Verification items for this drawing (mm, ordinates from the low corner). A direction names the side the tool comes from. Give positions to 0.01 mm unless a question says otherwise; leave off trailing zeros. Loops run counter-clockwise (first coordinate to the right, second up) from the corner with the lowest first, then second, coordinate; pieces in that order, holes last. Notation, with made-up numbers: (40.25, 65.5) -> (72.25, 65.5) arc R6 cw to (72.25, 73.5) -> close; hole circle Ø2 at (20.25, 49). An arc over 180 degrees is marked (long way). Answer as a JSON object with one key per item and string values.
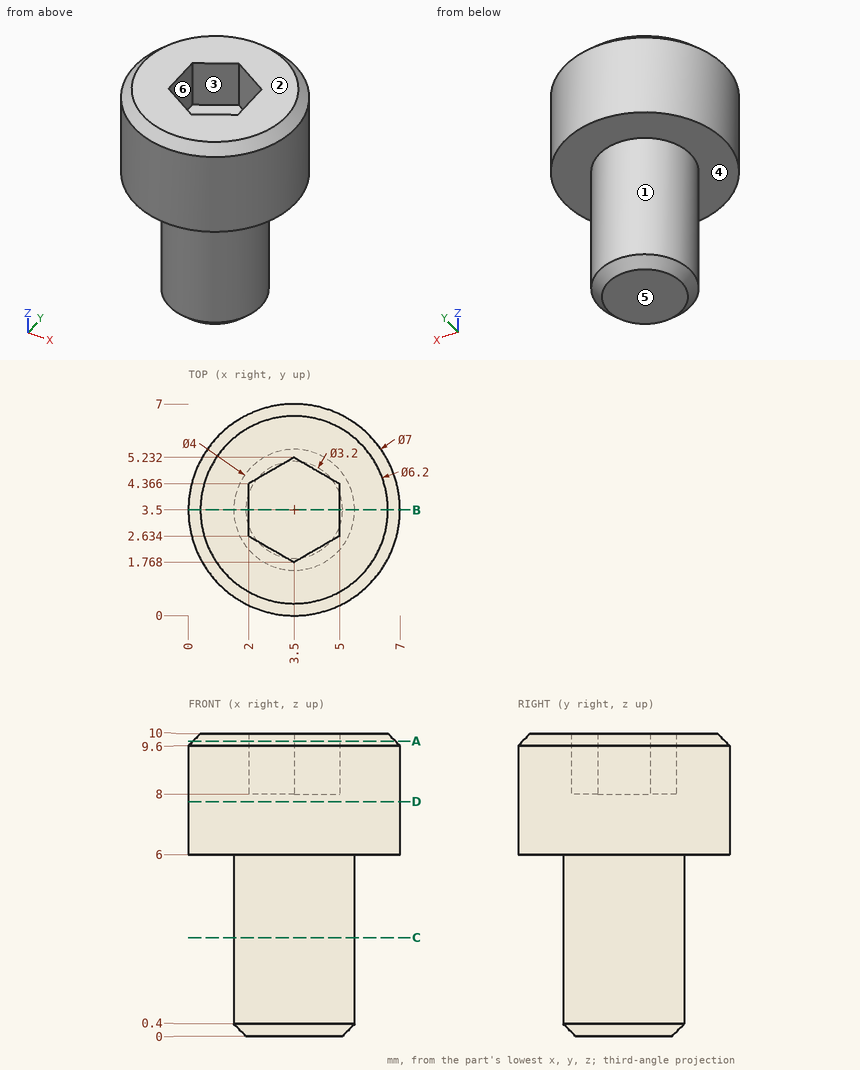
1) Draft check along X on the marked faces 1, 2 and 3. Enter one of: pulls with the +X half, pulls with the -X half, needs draft (parallel to the pull), parting line crosses it, or undercut.
Geometry check:
{"face 1": "parting line crosses it", "face 2": "needs draft", "face 3": "undercut"}
2) Section check C-C on z = 3.25. Record the cut outline in (x, y).
Geometry check:
{"outline": "circle Ø4 at (3.5, 3.5)"}
3) Depth check by flat-ended pin: P1, Ø0.5, axis at y = 4, z = 9, coming from the -X side; P2, Ø3, axis at x = 3, y = 5, coming from the -Z side; P3, Ø2, axis at x = 5.5, z = 9, coming from the -Y side. Enter the tip coordinate at first touch or a pass-through.
Geometry check:
{"P1": "stops at x = 0.01", "P2": "stops at z = 0", "P3": "stops at y = 0.15"}
4) Section check A-A on z = 9.75. Record the cut outline in (x, y).
Geometry check:
{"outline": "circle Ø6.7 at (3.5, 3.5); hole (2, 2.63) -> (3.5, 1.77) -> (5, 2.63) -> (5, 4.37) -> (3.5, 5.23) -> (2, 4.37) -> close"}
5) Tool access check on the marked faces 4, 5 and 6. Record the directions out of +Z, -Z, +X, -X, +Y, -Y that give a thin tool (end or side, any length) a straight path to the whole face; none if there is none.
Geometry check:
{"face 4": "-Z", "face 5": "-Z, +X, -X, +Y, -Y", "face 6": "+Z"}
6) Material ranges on line 1 along Z through (x, y) = (4, 6.25); line 2 along Y through (x, z) = (3.5, 3.25); line 3 along Z through (x, y) = (4.5, 4.5), recorded low to high. Write a range as from..to.
Geometry check:
{"line 1": "z = 6..10", "line 2": "y = 1.5..5.5", "line 3": "z = 0..8"}
7) Section check D-D on z = 7.75. Record the cut outline in (x, y).
Geometry check:
{"outline": "circle Ø7 at (3.5, 3.5)"}
8) Section check B-B on y = 3.5. Record the cut outline in (x, z).
Geometry check:
{"outline": "(0, 6) -> (1.5, 6) -> (1.5, 0.4) -> (1.9, 0) -> (5.1, 0) -> (5.5, 0.4) -> (5.5, 6) -> (7, 6) -> (7, 9.6) -> (6.6, 10) -> (5, 10) -> (5, 8) -> (2, 8) -> (2, 10) -> (0.4, 10) -> (0, 9.6) -> close"}
